The figure shows three views and two pictorial views of one solid part (mm, origin at its lowest corner). Answer the questions. A direction names the side the tool comes from. Round coordinates to 2 decimals unless told otherwise and drop trailing zeros. Order: outer loops, then holes, each group sorted by start corner. A loop starts at its lowest first (then second) coordinate and runs counter-clockwise, first axis right, second up. Notation, with made-up numbers: (22, 59.5) - (54, 59.5) arc R36 ccw to (54, 96.5) - close; hole circle Ø6 at (73, 66). An arc over 180 degrees is marked (long way). Answer in a Markdown table with one row per item.
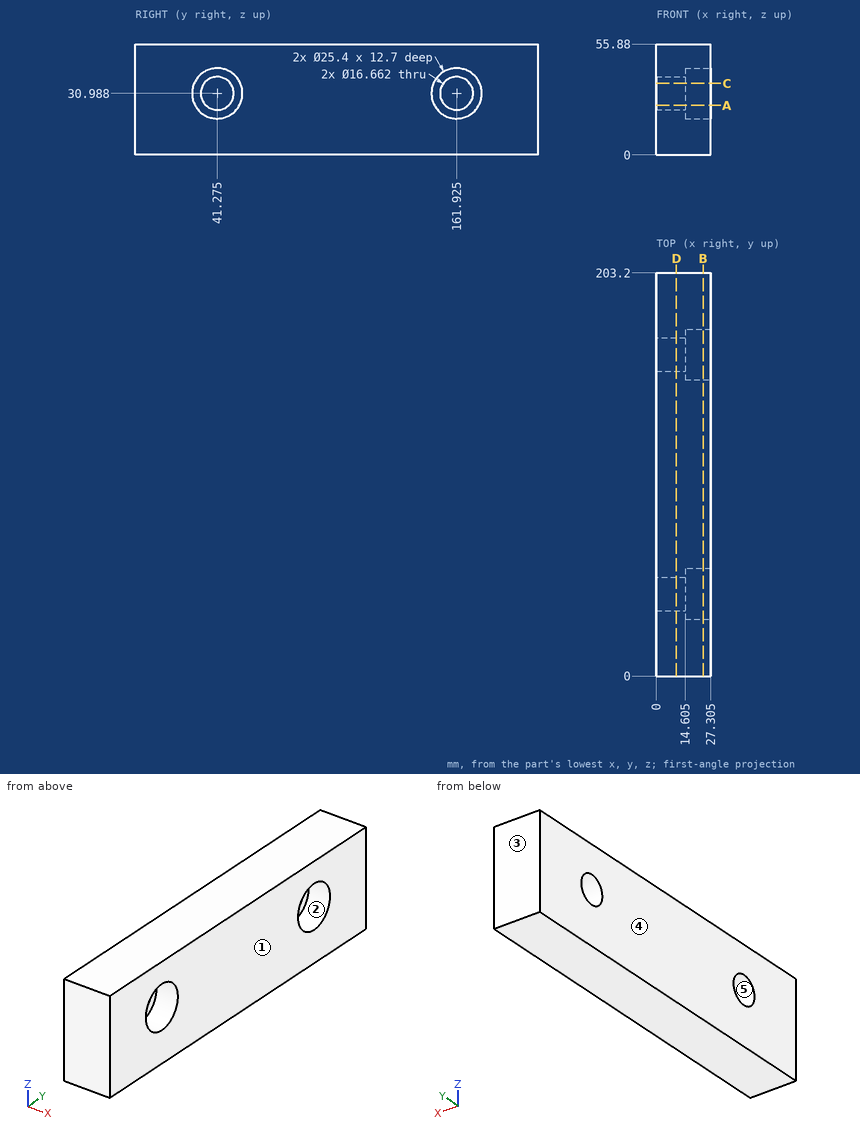
1) Find section B-B, the plane x = 23.5. Give the vertices of the cut face in (y, z) (1 decimal), then the cut area to 3 significant figures.
Filled in:
| item | result |
|---|---|
| outline | (0, 0) - (203.2, 0) - (203.2, 55.9) - (0, 55.9) - close; hole circle Ø25.4 at (41.3, 31); hole circle Ø25.4 at (161.9, 31) |
| area | 10,300 mm^2 |
2) The mould has two halves that part along Y. Classify the marked faces 3, 4 and 5: released by +Y, released by -Y, zero draft, split by the parting line, or undercut.
Filled in:
| item | result |
|---|---|
| face 3 | released by +Y |
| face 4 | zero draft |
| face 5 | undercut |
3) Which of the six approach directions +Z, -Z, +X, -X, +Y, -Y give full straight-line access (tool end or side, diameter ignored) to the marked faces 1 and 2?
Filled in:
| item | result |
|---|---|
| face 1 | +Z, -Z, +X, +Y, -Y |
| face 2 | +X |
4) Find section D-D, the plane x = 10. Give the vertices of the cut face in (y, z) (1 decimal).
Filled in:
| item | result |
|---|---|
| outline | (0, 0) - (203.2, 0) - (203.2, 55.9) - (0, 55.9) - close; hole circle Ø16.7 at (41.3, 31); hole circle Ø16.7 at (161.9, 31) |
5) Find the intervals of material crossed by probe 1 along Y at (x, z) = (11.25, 31.5); probe 2 along Y at (x, z) = (5, 35) (1 decimal), in increasing order. Write a range as from..to.
Filled in:
| item | result |
|---|---|
| probe 1 | y = 0..32.96, 49.59..153.61, 170.24..203.2 |
| probe 2 | y = 0..34, 48.6..154.6, 169.2..203.2 |
6) Find section C-C, the plane z = 36. Give the vertices of the cut face in (x, y) (1 decimal), then the cut area to 3 significant figures.
Filled in:
| item | result |
|---|---|
| outline | (0, 0) - (27.3, 0) - (27.3, 29.6) - (14.6, 29.6) - (14.6, 34.6) - (0, 34.6) - close; (0, 47.9) - (14.6, 47.9) - (14.6, 52.9) - (27.3, 52.9) - (27.3, 150.3) - (14.6, 150.3) - (14.6, 155.3) - (0, 155.3) - close; (0, 168.6) - (14.6, 168.6) - (14.6, 173.6) - (27.3, 173.6) - (27.3, 203.2) - (0, 203.2) - close |
| area | 4,570 mm^2 |
7) Each of these flat-tipped pins is pushed along its axis until it touches: pin 1 (1 mm diameter, centred on y = 172, z = 31, fed in from +X) (3 decimals); pin 2 (1 mm diameter, centred on y = 35, z = 34.5, fed in from +X). Where does it stop, or does it pass through?
Filled in:
| item | result |
|---|---|
| pin 1 | stops at x = 14.605 |
| pin 2 | passes through |
8) Find section A-A, the plane z = 25. Give the vertices of the cut face in (x, y) (1 decimal), then the cut area to 3 significant figures.
Filled in:
| item | result |
|---|---|
| outline | (0, 0) - (27.3, 0) - (27.3, 30.1) - (14.6, 30.1) - (14.6, 35.5) - (0, 35.5) - close; (0, 47.1) - (14.6, 47.1) - (14.6, 52.5) - (27.3, 52.5) - (27.3, 150.7) - (14.6, 150.7) - (14.6, 156.1) - (0, 156.1) - close; (0, 167.7) - (14.6, 167.7) - (14.6, 173.1) - (27.3, 173.1) - (27.3, 203.2) - (0, 203.2) - close |
| area | 4,640 mm^2 |
